from build123d import *

# Parameters (mm, degrees)
F0_R     = 2.15265
F1_DEPTH = 6.17728
F2_SIZE  = 4.7625


with BuildPart() as f1:
    # F0 (on Top) → F1 (new body)
    with BuildSketch(Plane.XY):
        with BuildLine():
            ThreePointArc((-14.5415, -8.55411), (-11.3665, -11.72911), (-14.5415, -14.90411))
            Line((-14.5415, -14.90411), (-14.5415, -28.86075))
            Line((-14.5415, -28.86075), (14.5415, -28.86075))
            Line((14.5415, -28.86075), (14.5415, -14.90411))
            ThreePointArc((14.5415, -14.90411), (11.3665, -11.72911), (14.5415, -8.55411))
            Line((14.5415, -8.55411), (14.5415, 28.86075))
            Line((14.5415, 28.86075), (-14.5415, 28.86075))
            Line((-14.5415, 28.86075), (-14.5415, -8.55411))
        make_face()
        with Locations((-4.8895, -24.892)):
            Circle(F0_R, mode=Mode.SUBTRACT)
        with Locations((4.8895, -24.892)):
            Circle(F0_R, mode=Mode.SUBTRACT)
        with Locations((-4.8895, 24.892)):
            Circle(F0_R, mode=Mode.SUBTRACT)
        with BuildLine():
            Line((9.779, 20.32), (9.779, -20.32))
            Line((9.779, -20.32), (1.016, -20.32))
            Line((1.016, -20.32), (1.016, -23.749))
            ThreePointArc((1.016, -23.749), (0, -24.765), (-1.016, -23.749))
            Line((-1.016, -23.749), (-1.016, -20.32))
            Line((-1.016, -20.32), (-9.779, -20.32))
            Line((-9.779, -20.32), (-9.779, 20.32))
            Line((-9.779, 20.32), (-1.016, 20.32))
            Line((-1.016, 20.32), (-1.016, 23.749))
            ThreePointArc((-1.016, 23.749), (0, 24.765), (1.016, 23.749))
            Line((1.016, 23.749), (1.016, 20.32))
            Line((1.016, 20.32), (9.779, 20.32))
        make_face(mode=Mode.SUBTRACT)
        with Locations((4.8895, 24.892)):
            Circle(F0_R, mode=Mode.SUBTRACT)
    extrude(amount=F1_DEPTH)

    # F2
    f2_edges = [f1.edges().sort_by_distance(p)[0] for p in [
        (14.5415, -28.86075, 3.08864),
        (14.5415, 28.86075, 3.08864),
        (-14.5415, 28.86075, 3.08864),
        (-14.5415, -28.86075, 3.08864),
    ]]
    chamfer(f2_edges, length=F2_SIZE)


solid = f1.part
Work out the finished part from the listing and answer in its coordinate system (mm). A direction names the side the tool comes from. Coordinates: 2 decimals unless noted, no trailing zeros. Loops run counter-clockwise (first coordinate to the right, second up) from the corner with the lowest first, then second, coordinate; pieces in that order, holes last. Notation, with made-up numbers: (37, -34) -> (83, -34) arc R18 cw to (83, -27) -> close; hole circle Ø5 at (-19.5, 60). An arc over 180 degrees is marked (long way). Answer as CSV lines item,"result".
1) The part is cut by section B-B (x = 0). Give the vertices of the cut face in (y, z) (3 decimals), and give its area (3 significant figures).
A:
outline,"(-28.861, 0) -> (-24.765, 0) -> (-24.765, 6.177) -> (-28.861, 6.177) -> close; (24.765, 0) -> (28.861, 0) -> (28.861, 6.177) -> (24.765, 6.177) -> close"
area,"50.6 mm²"
2) The part is cut by section C-C (x = 4). Give the vertices of the cut face in (y, z), and give its area (3 significant figures).
A:
outline,"(-28.86, 0) -> (-26.85, 0) -> (-26.85, 6.18) -> (-28.86, 6.18) -> close; (-22.93, 0) -> (-20.32, 0) -> (-20.32, 6.18) -> (-22.93, 6.18) -> close; (20.32, 0) -> (22.93, 0) -> (22.93, 6.18) -> (20.32, 6.18) -> close; (26.85, 0) -> (28.86, 0) -> (28.86, 6.18) -> (26.85, 6.18) -> close"
area,"57.1 mm²"
3) Straight lines are drawn through the part: probe 1 along X at (y, z) = (14, 4.5); probe 2 along Y at (x, z) = (1.75, 4.5); probe 3 along X at (y, z) = (-25.5, 1.25). For each, find the intervals that lie inside material, in ascending order.
A:
probe 1,"x = -14.54 to -9.78, 9.78 to 14.54"
probe 2,"y = -28.86 to -20.32, 20.32 to 28.86"
probe 3,"x = -13.14 to -6.95, -2.82 to 2.82, 6.95 to 13.14"
4) The part is cut by section A-A (y = -2). Give the vertices of the cut face in (x, z), and give its area (3 significant figures).
A:
outline,"(-14.54, 0) -> (-9.78, 0) -> (-9.78, 6.18) -> (-14.54, 6.18) -> close; (9.78, 0) -> (14.54, 0) -> (14.54, 6.18) -> (9.78, 6.18) -> close"
area,"58.8 mm²"
5) The part is cut by section D-D (z = 5). State how many separate pieces and enclosed holes the cut face has, and give its area (3 significant figures).
A:
separate pieces,"1"
enclosed holes,"5"
area,"731 mm²"
6) For a pull along Y with two mould halves and no side action, classify faces 1 (the face through (1.016, -22, 3)), 2 (the face through (11, 2, 0)), 3 (the face through (-12.13, 26.51, 3.05)) as released by +Y, released by -Y, zero draft, split by the parting line, or undercut.
A:
face 1,"undercut"
face 2,"zero draft"
face 3,"released by +Y"
7) A flat-ended cylindrical pin translates along its axis: pin 1 (2.5 mm diameter, centred on x = -4.89, y = 24.89, fed in from +Z). Find the tip coordinate at first contact, or state that the pin passes through.
A:
pin 1,"passes through"
8) For faces 4 (the face through (11, 2, 6.177)), 5 (the face through (-5, -20.32, 3)), determine the directions among +Z, -Z, +X, -X, +Y, -Y from which every point of the face is accessible in a straight line to the end or side of a thin tool.
A:
face 4,"+Z, +X, -X, +Y, -Y"
face 5,"+Z, -Z"
